Autodesk Inventor part; units mm, degrees
ref_plane "YZ Plane" through (0, 0, 0) normal (1, 0, 0) x (0, 1, 0)
ref_plane "XZ Plane" through (0, 0, 0) normal (0, 1, 0) x (-1, 0, 0)
ref_plane "XY Plane" through (0, 0, 0) normal (0, 0, 1) x (1, 0, 0)
ref_plane "Work Plane1" through (0, 0, 19.05) normal (0, 0, 1) x (1, 0, 0)
sketch "Sketch2" plane through (0, 0, 19.05) normal (0, 0, 1) x (1, 0, 0)
  line L0 (1453.4656, 254.6366) -> (-578.5344, 254.6366)
  line L1 (-578.5344, 254.6366) -> (-559.4844, 254.6366)
  line L2 (-559.4844, -151.7634) -> (-578.5344, -151.7634)
  line L3 (-578.5344, -151.7634) -> (-578.5344, 254.6366)
  line L4 (1453.4656, -151.7634) -> (1453.4656, 254.6366)
  line L5 (-578.5344, -151.7634) -> (1453.4656, -151.7634)
  line L6 (1453.4656, 254.6366) -> (1434.4156, 254.6366)
  line L7 (1434.4156, -151.7634) -> (1453.4656, -151.7634)
  line L8 (1453.4656, -151.7634) -> (1453.4656, 254.6366)
  line L9 (-578.5344, 254.6366) -> (-578.5344, -151.7634)
  line L10 (-559.4844, 254.6366) -> (-559.4844, 203.8366)
  line L11 (-578.5344, 203.8366) -> (-559.4844, 203.8366)
  line L12 (1434.4156, 203.8366) -> (1453.4656, 203.8366)
  line L13 (-578.5344, 102.2366) -> (-559.4844, 102.2366)
  line L14 (1434.4156, 102.2366) -> (1453.4656, 102.2366)
  line L15 (-578.5344, 0.6366) -> (-559.4844, 0.6366)
  line L16 (1434.4156, 0.6366) -> (1453.4656, 0.6366)
  line L17 (-578.5344, -100.9634) -> (-559.4844, -100.9634)
  line L18 (1434.4156, -100.9634) -> (1453.4656, -100.9634)
  line L19 (-559.4844, 102.2366) -> (-559.4844, 0.6366)
  line L20 (-559.4844, -100.9634) -> (-559.4844, -151.7634)
  line L21 (1434.4156, 254.6366) -> (1434.4156, 203.8366)
  line L22 (1434.4156, 102.2366) -> (1434.4156, 0.6366)
  line L23 (1434.4156, -100.9634) -> (1434.4156, -151.7634)
  line L24 (-578.5344, 254.6366) -> (-559.4844, 254.6366)
  line L25 (-559.4844, 254.6366) -> (-559.4844, 203.8366)
  line L26 (-559.4844, 203.8366) -> (-578.5344, 203.8366)
  line L27 (-578.5344, 203.8366) -> (-578.5344, 254.6366)
  line L28 (-578.5344, 102.2366) -> (-559.4844, 102.2366)
  line L29 (-559.4844, 102.2366) -> (-559.4844, 0.6366)
  line L30 (-559.4844, 0.6366) -> (-578.5344, 0.6366)
  line L31 (-578.5344, 0.6366) -> (-578.5344, 102.2366)
  line L32 (-578.5344, -100.9634) -> (-559.4844, -100.9634)
  line L33 (-559.4844, -100.9634) -> (-559.4844, -151.7634)
  line L34 (-559.4844, -151.7634) -> (-578.5344, -151.7634)
  line L35 (-578.5344, -151.7634) -> (-578.5344, -100.9634)
  line L36 (1453.4656, 254.6366) -> (1434.4156, 254.6366)
  line L37 (1434.4156, 254.6366) -> (1434.4156, 203.8366)
  line L38 (1434.4156, 203.8366) -> (1453.4656, 203.8366)
  line L39 (1453.4656, 203.8366) -> (1453.4656, 254.6366)
  line L40 (1453.4656, 102.2366) -> (1434.4156, 102.2366)
  line L41 (1434.4156, 102.2366) -> (1434.4156, 0.6366)
  line L42 (1434.4156, 0.6366) -> (1453.4656, 0.6366)
  line L43 (1453.4656, 0.6366) -> (1453.4656, 102.2366)
  line L44 (1453.4656, -100.9634) -> (1434.4156, -100.9634)
  line L45 (1434.4156, -100.9634) -> (1434.4156, -151.7634)
  line L46 (1434.4156, -151.7634) -> (1453.4656, -151.7634)
  line L47 (1453.4656, -151.7634) -> (1453.4656, -100.9634)
  point P0 (0, 0)
extrude "Extrusion2" add sketch "Sketch2" along normal blind 19.05 contours L21 L12 L4 L14 L22 L16 L18 L23 L5 L20 L17 L3 L15 L19 L13 L11 L10 L0
sketch "Sketch3" plane through (0, 0, 38.1) normal (0, 0, 1) x (1, 0, 0)
  line L0 (1434.4156, 254.6366) -> (-559.4844, 254.6366)
  line L1 (1453.4656, 102.2366) -> (1453.4656, 203.8366)
  line L2 (-559.4844, -151.7634) -> (1434.4156, -151.7634)
  line L3 (-559.4844, 254.6366) -> (-426.1344, 254.6366)
  line L4 (-559.4844, 235.5866) -> (-426.1344, 235.5866)
  line L5 (-222.9344, 254.6366) -> (-121.3344, 254.6366)
  line L6 (-222.9344, 235.5866) -> (-121.3344, 235.5866)
  line L7 (81.8656, 254.6366) -> (183.4656, 254.6366)
  line L8 (81.8656, 235.5866) -> (183.4656, 235.5866)
  line L9 (386.6656, 254.6366) -> (488.2656, 254.6366)
  line L10 (386.6656, 235.5866) -> (488.2656, 235.5866)
  line L11 (691.4656, 254.6366) -> (793.0656, 254.6366)
  line L12 (691.4656, 235.5866) -> (793.0656, 235.5866)
  line L13 (996.2656, 254.6366) -> (1097.8656, 254.6366)
  line L14 (1301.0656, 254.6366) -> (1434.4156, 254.6366)
  line L15 (996.2656, 235.5866) -> (1097.8656, 235.5866)
  line L16 (1301.0656, 235.5866) -> (1434.4156, 235.5866)
  line L17 (1301.0656, 254.6366) -> (1301.0656, 235.5866)
  line L18 (1301.0656, -132.7134) -> (1301.0656, -151.7634)
  line L19 (1097.8656, 254.6366) -> (1097.8656, 235.5866)
  line L20 (1097.8656, -132.7134) -> (1097.8656, -151.7634)
  line L21 (996.2656, 254.6366) -> (996.2656, 235.5866)
  line L22 (996.2656, -132.7134) -> (996.2656, -156.6063)
  line L23 (793.0656, 254.6366) -> (793.0656, 235.5866)
  line L24 (793.0656, -132.7134) -> (793.0656, -151.7634)
  line L25 (691.4656, 254.6366) -> (691.4656, 235.5866)
  line L26 (691.4656, -132.7134) -> (691.4656, -151.7634)
  line L27 (488.2656, 254.6366) -> (488.2656, 235.5866)
  line L28 (488.2656, -132.7134) -> (488.2656, -151.7634)
  line L29 (386.6656, 254.6366) -> (386.6656, 235.5866)
  line L30 (386.6656, -132.7134) -> (386.6656, -151.7634)
  line L31 (183.4656, 254.6366) -> (183.4656, 235.5866)
  line L32 (183.4656, -132.7134) -> (183.4656, -151.7634)
  line L33 (81.8656, 254.6366) -> (81.8656, 235.5866)
  line L34 (81.8656, -132.7134) -> (81.8656, -151.7634)
  line L35 (-121.3344, 254.6366) -> (-121.3344, 235.5866)
  line L36 (-121.3344, -132.7134) -> (-121.3344, -156.6063)
  line L37 (-222.9344, 254.6366) -> (-222.9344, 235.5866)
  line L38 (-222.9344, -132.7134) -> (-222.9344, -151.7634)
  line L39 (-426.1344, 254.6366) -> (-426.1344, 235.5866)
  line L40 (-426.1344, -132.7134) -> (-426.1344, -151.7634)
  line L41 (-426.1344, -132.7134) -> (-559.4844, -132.7134)
  line L42 (-559.4844, -132.7134) -> (-426.1344, -132.7134)
  line L43 (-426.1344, -151.7634) -> (-559.4844, -151.7634)
  line L44 (-121.3344, -132.7134) -> (-222.9344, -132.7134)
  line L45 (-121.3344, -151.7634) -> (-222.9344, -151.7634)
  line L46 (-222.9344, -132.7134) -> (-121.3344, -132.7134)
  line L47 (183.4656, -151.7634) -> (81.8656, -151.7634)
  line L48 (183.4656, -132.7134) -> (81.8656, -132.7134)
  line L49 (81.8656, -132.7134) -> (183.4656, -132.7134)
  line L50 (488.2656, -132.7134) -> (386.6656, -132.7134)
  line L51 (488.2656, -151.7634) -> (386.6656, -151.7634)
  line L52 (386.6656, -132.7134) -> (488.2656, -132.7134)
  line L53 (793.0656, -132.7134) -> (691.4656, -132.7134)
  line L54 (793.0656, -151.7634) -> (691.4656, -151.7634)
  line L55 (691.4656, -132.7134) -> (793.0656, -132.7134)
  line L56 (1434.4156, -132.7134) -> (1301.0656, -132.7134)
  line L57 (1097.8656, -132.7134) -> (996.2656, -132.7134)
  line L58 (1434.4156, -151.7634) -> (1301.0656, -151.7634)
  line L59 (1097.8656, -151.7634) -> (996.2656, -151.7634)
  line L60 (996.2656, -132.7134) -> (1097.8656, -132.7134)
  line L61 (1301.0656, -132.7134) -> (1434.4156, -132.7134)
  line L62 (1434.4156, 254.6366) -> (1434.4156, 235.5866)
  line L63 (1434.4156, -132.7134) -> (1434.4156, -151.7634)
  line L64 (-559.4844, 254.6366) -> (-559.4844, 235.5866)
  line L65 (-559.4844, -132.7134) -> (-559.4844, -151.7634)
  point P0 (0, 0)
  point P1 (1453.4656, -132.7134)
  point P2 (1545.8427, 235.5866)
  point P3 (874.9313, 0)
extrude "Extrusion3" cut sketch "Sketch3" against normal blind 19.05
properties part number "bottom" material "Wood (Birch)"
Can you work these out from the model? Positions are in its coordinate system, mm. Give positions to 0.01 mm unless a question says otherwise; leave off trailing zeros. Loops run counter-clockwise (first coordinate to the right, second up) from the corner with the lowest first, then second, coordinate; pieces in that order, holes last. Notation, with made-up numbers: (85.5, 37) - (126.5, 37) arc R22 cw to (126.5, 52) - close; hole circle Ø6 at (10, 65). An arc over 180 degrees is marked (long way). One line per item, written item: value.
(1) If we section it at A-A, the plane y = 56: List the corners of the cut face in (x, z) for me, plus the area to 3 significant figures.
Verdict:
outline: (-559.48, 19.05) - (1434.42, 19.05) - (1434.42, 38.1) - (-559.48, 38.1) - close
area: 38,000 mm^2
(2) I'm going to push flat-ended pins straight in: pin 1 (9.5 mm diameter, centred on x = 1045, z = 26, fed in from +Y); pin 2 (9.5 mm diameter, centred on y = 244.5, z = 30.5, fed in from +X); pin 3 (5.5 mm diameter, centred on y = -141.5, z = 27, fed in from -X). Where does each tip first touch, or does it pass through?
Verdict:
pin 1: y = 235.59
pin 2: x = 1301.07
pin 3: x = -426.13
(3) I need wall thicknesses on line 1 along X through (y, z) = (88, 21.75); line 2 along Y through (x, z) = (1018, 20). Which ranges of each line are inside material? Lowest first, please.
Verdict:
line 1: -559.48 to 1434.42
line 2: -132.71 to 235.59
(4) If we section it at B-B, the plane x = -188: List the corners of the cut face in (y, z) for me, plus the area to 3 significant figures.
Verdict:
outline: (-132.71, 19.05) - (235.59, 19.05) - (235.59, 38.1) - (-132.71, 38.1) - close
area: 7,020 mm^2
